from build123d import *

# Parameters (mm, degrees)
RESSALTO_EXTRUS_O1_DEPTH = 35
ESBO_O2_R                = 1.5
CORTE_EXTRUS_O1_DEPTH    = 8
CORTE_EXTRUS_O2_START    = -8
ESBO_O3_R                = 1.5
CORTE_EXTRUS_O2_DEPTH    = 8


with BuildPart() as part:
    # Esboço1 → Ressalto-extrusão1 (new body)
    with BuildSketch(Plane(origin=(0, 0, 0), x_dir=(1, 0, 0), z_dir=(0, 1, 0))):
        Polygon((2.5, 0), (1.25, 2.165063509), (-1.25, 2.165063509), (-2.5, 0), (-1.25, -2.165063509), (1.25, -2.165063509), align=None)
    extrude(amount=RESSALTO_EXTRUS_O1_DEPTH)

    # Esboço2 → Corte-extrusão1 (cut)
    with BuildSketch(Plane(origin=(0, 35, 0), x_dir=(1, 0, 0), z_dir=(0, 1, 0))):
        with Locations(Location((0, 0, 0), (0, 0, 270))):
            Circle(ESBO_O2_R)
    extrude(amount=-CORTE_EXTRUS_O1_DEPTH, mode=Mode.SUBTRACT)

    # Esboço3 → Corte-extrusão2 (cut)
    with BuildSketch(Plane.XZ.offset(CORTE_EXTRUS_O2_START)):
        with Locations(Location((0, 0, 0), (0, 0, 90))):
            Circle(ESBO_O3_R)
    extrude(amount=CORTE_EXTRUS_O2_DEPTH, mode=Mode.SUBTRACT)


solid = part.part
Can you work these out from the model? Positions are in its coordinate system, mm. A direction names the side the tool comes from. Round coordinates to 2 decimals unless told otherwise and drop trailing zeros. Loops run counter-clockwise (first coordinate to the right, second up) from the corner with the lowest first, then second, coordinate; pieces in that order, holes last. Notation, with made-up numbers: (54, -39.5) - (93, -39.5) arc R21 ccw to (93, -10.5) - close; hole circle Ø1 at (17.5, -25). An arc over 180 degrees is marked (long way). Write item = value, one per line. Start each with the question number.
(1) If we section it at A-A (y = 6): Please give me the cut outline in (x, z).
(2) If we section it at B-B (x = 0): Please give me the cut outline in (y, z), and give its area (3 significant figures).
(3) If I drill on probe 1 along Y at (x, z) = (1.1, -0.8); probe 2 along X at (y, z) = (6.5, 0.8); probe 3 along Z at (x, y) = (-1.3, 3.5), over which ranges is the centre line in solid material (lowest first)? Write a range as [from, to].
(4) If we section it at C-C (z = 0.45): Please give me the cut outline in (x, y), and give its area (3 significant figures).
(5) For faces 5 (the face through (-1.866, 17.255, -1.098)), 6 (the face through (0, 8, 0)), 7 (the face through (0.45, 31.06, 1.43)), which set-ups out of +Z, -Z, +X, -X, +Y, -Y let a thin tool reach every point of the face, with its end or its side?
(6) If we section it at D-D (y = 11): Please give me the cut outline in (x, z).
(7) For P1, Ø2.5, axis at x = 0, z = 0, coming from the +Y side; P2, Ø1.5, axis at x = 0, z = 0, coming from the -Y side, each with a flat end and sliding along its axis, tell me the tip position at first contact or that it passes through.
(8) If we mould it in two halves opening along Z, with no side actions, what happens to faces 1 (the face through (0, 17, 2.165)), 2 (the face through (0, 27, 0)), 3 (the face through (2, 35, 0)), 4 (the face through (0, 17, -2.165))? For each: released by +Z, released by -Z, zero draft, split by the parting line, or undercut.
Ans:
q1.outline = (-2.5, 0) - (-1.25, -2.17) - (1.25, -2.17) - (2.5, 0) - (1.25, 2.17) - (-1.25, 2.17) - close; hole circle Ø3 at (0, 0)
q2.outline = (0, -2.17) - (35, -2.17) - (35, -1.5) - (27, -1.5) - (27, 1.5) - (35, 1.5) - (35, 2.17) - (0, 2.17) - (0, 1.5) - (8, 1.5) - (8, -1.5) - (0, -1.5) - close
q2.area = 104 mm²
q3.probe_1 = [8, 27]
q3.probe_2 = [-2.04, -1.27], [1.27, 2.04]
q3.probe_3 = [-2.08, -0.75], [0.75, 2.08]
q4.outline = (-2.24, 0) - (-1.43, 0) - (-1.43, 8) - (1.43, 8) - (1.43, 0) - (2.24, 0) - (2.24, 35) - (1.43, 35) - (1.43, 27) - (-1.43, 27) - (-1.43, 35) - (-2.24, 35) - close
q4.area = 111 mm²
q5.face_5 = -Z, -X, +Y, -Y
q5.face_6 = -Y
q5.face_7 = +Y
q6.outline = (-2.5, 0) - (-1.25, -2.17) - (1.25, -2.17) - (2.5, 0) - (1.25, 2.17) - (-1.25, 2.17) - close
q7.P1 = 27
q7.P2 = 8
q8.face_1 = released by +Z
q8.face_2 = undercut
q8.face_3 = zero draft
q8.face_4 = released by -Z
